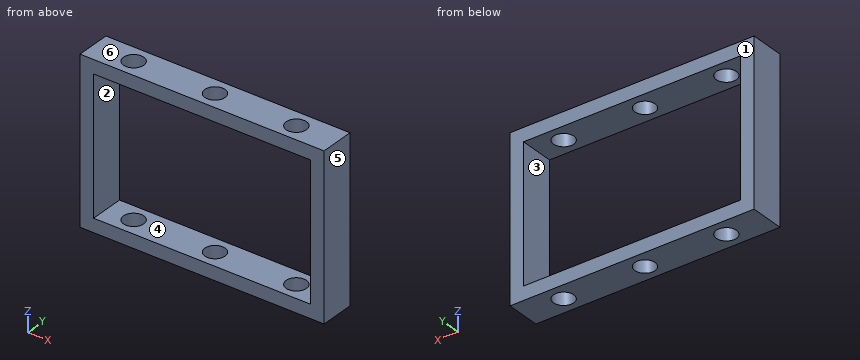
from build123d import *

# Parameters (mm, degrees)
F0_W     = 90
F0_H     = 60
F0_W_2   = 80
F0_H_2   = 50
F1_DEPTH = 12.7
F2_R     = 3.75
F3_DEPTH = 76.2


# Not quite as in the source:
# - a feature names something its author has since deleted; it is built from what else it names


with BuildPart() as f1:
    # F0 (on Front) → F1 (new body)
    with BuildSketch(Plane.XZ):
        Rectangle(F0_W, F0_H)
        Rectangle(F0_W_2, F0_H_2, mode=Mode.SUBTRACT)
    extrude(amount=F1_DEPTH)

    # F2 (on face) → F3 (cut)
    with BuildSketch(Plane(origin=(0, 0, -30), x_dir=(1, 0, 0), z_dir=(0, 0, -1))):
        with Locations((-30, 6.35)):
            Circle(F2_R)
        with Locations((0, 6.35)):
            Circle(F2_R)
        with Locations((30, 6.35)):
            Circle(F2_R)
    extrude(amount=-F3_DEPTH, mode=Mode.SUBTRACT)


solid = f1.part
For this review, take the finished solid that the model builds, in its own axes (mm). Face numbers are marked on the shaded views. A direction names the side the tool comes from. Coordinates: 2 decimals unless noted, no trailing zeros. Order: outer loops, then holes, each group sorted by start corner. A loop starts at its lowest first (then second) coordinate and runs counter-clockwise, first axis right, second up. Notation, with made-up numbers: (46.25, 68.5) - (97.25, 68.5) arc R14 ccw to (97.25, 74.5) - close; hole circle Ø6 at (42, 20.5). An arc over 180 degrees is marked (long way). Use one line per item in the form item = value.
Q1. Consider section A-A (z = 5). Give the boundary of the cut face in (x, y).
Checked values:
outline = (-45, -12.7) - (-40, -12.7) - (-40, 0) - (-45, 0) - close; (40, -12.7) - (45, -12.7) - (45, 0) - (40, 0) - close
Q2. Consider section D-D (y = -11.5). Give the boundary of the cut face in (x, z).
Checked values:
outline = (-45, -30) - (45, -30) - (45, 30) - (-45, 30) - close; hole (-40, -25) - (40, -25) - (40, 25) - (-40, 25) - close
Q3. For probe 1 along X at (y, z) = (-6.35, -27.35); probe 2 along Z at (x, y) = (-24.5, -0.25); probe 3 along Y at (x, z) = (0, -28.85), list the stretches that pass through material, from the lowest coordinate up. Write a range as from..to.
Checked values:
probe_1 = -45..-33.75, -26.25..-3.75, 3.75..26.25, 33.75..45
probe_2 = -30..-25, 25..30
probe_3 = -12.7..-10.1, -2.6..0
Q4. For P1, Ø7, axis at x = 30, y = -6.35, coming from the -Z side, flat-tipped, find the tip position at first contact; note if it passes through.
Checked values:
P1 = through
Q5. For the marked faces 1 and 2, list the 3-axis set-ups (+Z, -Z, +X, -X, +Y, -Y) from which the entire face can be reached by the end or side of a thin tool; tool diameter is ignored.
Checked values:
face_1 = +Z, -Z, +X, -X, +Y
face_2 = +Y, -Y
Q6. Draft analysis for pull direction X (two halves, no side actions). For the marked faces 3, 4, 5 and 6, state which applies: +X half, -X half, draft (parallel to the pull), parting line (faces both ways), or undercut.
Checked values:
face_3 = undercut
face_4 = undercut
face_5 = +X half
face_6 = draft
Q7. Consider section B-B (y = -6.35). Give the number of separate pieces and of enclosed holes in the cut face, then the cut area to 4 significant figures.
Checked values:
separate_pieces = 6
enclosed_holes = 0
area = 1,175 mm2
Q8. Consider section C-C (x = 30). Give the boundary of the cut face in (y, z), then the cut area to 3 significant figures.
Checked values:
outline = (-12.7, -30) - (-10.1, -30) - (-10.1, -25) - (-12.7, -25) - close; (-12.7, 25) - (-10.1, 25) - (-10.1, 30) - (-12.7, 30) - close; (-2.6, -30) - (0, -30) - (0, -25) - (-2.6, -25) - close; (-2.6, 25) - (0, 25) - (0, 30) - (-2.6, 30) - close
area = 52.0 mm2
